The model under review builds one solid part; all positions refer to its coordinate system, in mm. Face numbers are marked on the shaded views. A direction names the side the tool comes from. Round coordinates to 2 decimals unless told otherwise and drop trailing zeros. Order: outer loops, then holes, each group sorted by start corner. A loop starts at its lowest first (then second) coordinate and runs counter-clockwise, first axis right, second up.
1) Consider section C-C (z = 5). Give the boundary of the cut face in (x, y), then the cut area to 3 significant figures.
2) Consider section D-D (x = -16). Give the boundary of the cut face in (y, z).
3) Machinability: for the marked faces 4 and 5, which of the approach directions +Z, -Z, +X, -X, +Y, -Y give a long, thin tool a straight path to every point of the face, cutting with its end or side? Answer none if there is none.
4) Consider section B-B (y = 11). Give the boundary of the cut face in (x, z), then the cut area to 3 significant figures.
5) Consider section A-A (x = 0). Give the boundary of the cut face in (y, z).
6) Clearance check with flat-ended pins moving along their axes: P1, Ø2, axis at y = -1, z = 25.5, coming from the +X side; P2, Ø8, axis at y = -8.5, z = 18.5, coming from the -X side; P3, Ø1.6, axis at y = 3.5, z = 28.5, coming from the +X side. State where each tip first meets the part, or that it passes through.
7) To check wall thickness, follow L1, parallel to Y at x = 0, z = 5; L2, parallel to Y at x = 0, z = 1.95; L3, parallel to Y at x = 16.5, z = 4.5. State the ranges of each line that lie inside material, in increasing order.
8) Mouldability with a two-part tool opening along X and no side actions: class the marked faces 1, 2 and 3 as pulls with the +X half, pulls with the -X half, needs draft (parallel to the pull), parting line crosses it, or undercut.
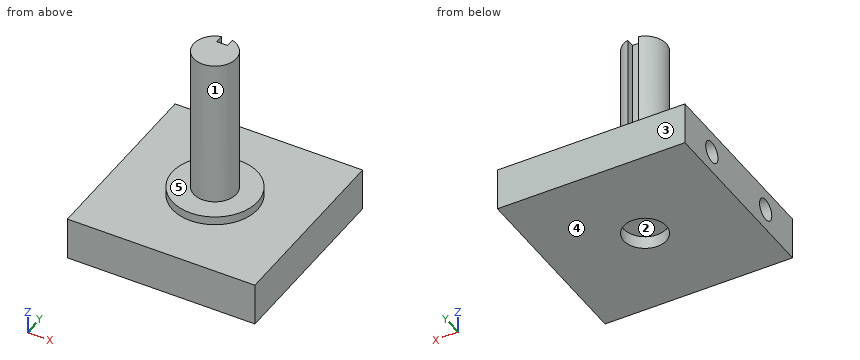
from build123d import *

# Parameters (mm, degrees)
SKETCH1_W           = 44
SKETCH1_H           = 44
BOSS_EXTRUDE1_DEPTH = 10
SKETCH2_R           = 5
BOSS_EXTRUDE2_DEPTH = 37
SKETCH3_R           = 5
BOSS_EXTRUDE3_DEPTH = 3
SKETCH4_R           = 5
CUT_EXTRUDE1_DEPTH  = 3
SKETCH5_R           = 2.5
CUT_EXTRUDE2_DEPTH  = 41
SKETCH6_R           = 10
BOSS_EXTRUDE4_DEPTH = 2
SKETCH7_W           = 2.5
SKETCH7_H           = 3
CUT_EXTRUDE3_DEPTH  = 30


with BuildPart() as part:
    # Sketch1 → Boss-Extrude1 (new body)
    with BuildSketch(Plane.XY):
        Rectangle(SKETCH1_W, SKETCH1_H)
    extrude(amount=BOSS_EXTRUDE1_DEPTH)

    # Sketch2 → Boss-Extrude2 (add)
    with BuildSketch(Plane.XY.offset(10)):
        Circle(SKETCH2_R)
    extrude(amount=BOSS_EXTRUDE2_DEPTH)

    # Sketch3 → Boss-Extrude3 (add)
    with BuildSketch(Plane(origin=(0, 0, 0), x_dir=(-1, 0, 0), z_dir=(0, 0, -1))):
        with Locations(Location((0, 0, 0), (0, 0, 180))):
            Circle(SKETCH3_R)
    extrude(amount=-BOSS_EXTRUDE3_DEPTH)

    # Sketch4 → Cut-Extrude1 (cut)
    with BuildSketch(Plane(origin=(0, 0, 0), x_dir=(-1, 0, 0), z_dir=(0, 0, -1))):
        with Locations(Location((0, 0, 0), (0, 0, 180))):
            Circle(SKETCH4_R)
    extrude(amount=-CUT_EXTRUDE1_DEPTH, mode=Mode.SUBTRACT)

    # Sketch5 → Cut-Extrude2 (cut)
    with BuildSketch(Plane.ZY.offset(22)):
        with Locations((5, -11)):
            Circle(SKETCH5_R)
        with Locations((5, 11)):
            Circle(SKETCH5_R)
    extrude(amount=-CUT_EXTRUDE2_DEPTH, mode=Mode.SUBTRACT)

    # Sketch6 → Boss-Extrude4 (add)
    with BuildSketch(Plane.XY.offset(10)):
        Circle(SKETCH6_R)
    extrude(amount=BOSS_EXTRUDE4_DEPTH)

    # Sketch7 → Cut-Extrude3 (cut)
    with BuildSketch(Plane.XY.offset(47)):
        with Locations((0, 4.385245902)):
            Rectangle(SKETCH7_W, SKETCH7_H)
    extrude(amount=-CUT_EXTRUDE3_DEPTH, mode=Mode.SUBTRACT)


solid = part.part
Answer below:
1. outline: (-22, -22) - (22, -22) - (22, 22) - (-22, 22) - (-22, 13.5) - (19, 13.5) - (19, 8.5) - (-22, 8.5) - (-22, -8.5) - (19, -8.5) - (19, -13.5) - (-22, -13.5) - close
1. area: 1,530 mm2
2. outline: (-22, 0) - (22, 0) - (22, 10) - (-22, 10) - close; hole circle Ø5 at (-11, 5); hole circle Ø5 at (11, 5)
3. face 4: -Z, +X, -X, +Y, -Y
3. face 5: +Z
4. outline: (-22, 0) - (22, 0) - (22, 10) - (-22, 10) - (-22, 7.5) - (19, 7.5) - (19, 2.5) - (-22, 2.5) - close
4. area: 235 mm2
5. outline: (-22, 0) - (-5, 0) - (-5, 3) - (5, 3) - (5, 0) - (22, 0) - (22, 10) - (10, 10) - (10, 12) - (5, 12) - (5, 17) - (2.89, 17) - (2.89, 47) - (-5, 47) - (-5, 12) - (-10, 12) - (-10, 10) - (-22, 10) - close; hole circle Ø5 at (-11, 5); hole circle Ø5 at (11, 5)
6. P1: stops at x = 5
6. P2: stops at x = -2.18
6. P3: stops at x = 4.21
7. L1: y = -22 to -13.5, -8.5 to 8.5, 13.5 to 22
7. L2: y = -22 to -5, 5 to 22
7. L3: y = -22 to -13.45, -8.55 to 8.55, 13.45 to 22
8. face 1: parting line crosses it
8. face 2: undercut
8. face 3: needs draft
